Autodesk Inventor part; units mm, degrees
ref_plane "YZ Plane" through (0, 0, 0) normal (1, 0, 0) x (0, 1, 0)
ref_plane "XZ Plane" through (0, 0, 0) normal (0, 1, 0) x (-1, 0, 0)
ref_plane "XY Plane" through (0, 0, 0) normal (0, 0, 1) x (1, 0, 0)
sketch "草图1" plane through (0, 0, 0) normal (0, 0, 1) x (1, 0, 0)
  line L0 (0, 0) -> (0, 15) construction
  line L1 (2.5, 0) -> (2.5, 15)
  line L2 (-2.5, 15) -> (-2.5, 0)
  arc A0 (-2.5, 0) -> (2.5, 0) centre (0, 0) ccw
  arc A1 (2.5, 15) -> (-2.5, 15) centre (0, 15) ccw
  point P0 (0, 7.5)
  point P1 (0, -2.5)
  point P2 (0, 17.5)
  dimension "d2" = 20
  dimension "d3" = 5
extrude "拉伸1" add sketch "草图1" along normal blind 2
sketch "草图2" plane through (0, 0, 2) normal (0, 0, 1) x (1, 0, 0)
  circle A0 centre (0, 0) radius 1.5
  arc A1 (2.5, 15) -> (-2.5, 15) centre (0, 15) ccw
  circle A2 centre (0, 15) radius 1.5
  dimension "d4" = 3
  dimension "d5" = 3
extrude "拉伸2" cut sketch "草图2" against normal blind 3
properties part number "连杆2"
Part model, mm, in its own coordinate system. Coordinates: 2 decimals unless noted, no trailing zeros. Loops run counter-clockwise (first coordinate to the right, second up) from the corner with the lowest first, then second, coordinate; pieces in that order, holes last. Notation, with made-up numbers: (22.25, 11) -> (45.25, 11) arc R11 ccw to (45.25, 22) -> close; hole circle Ø6 at (84.25, 1.25). An arc over 180 degrees is marked (long way). Use a Markdown table: item, result. Add a question column.
Item 1: Band-saw the part on C-C on z = 1.3. Write the cut outline in (x, y).
Item 2: Band-saw the part on A-A on x = 0. Write the cut outline in (y, z), plus the area to 3 significant figures.
Item 3: Flat gauge pins, fed straight in: P1, Ø2.5, axis at x = 0, y = 15, coming from the -Z side; P2, Ø1, axis at x = 2, y = 9.5, coming from the -Z side; P3, Ø1, axis at x = -2, z = 0.5, coming from the +Y side. Where does each tip first touch, or does it go through?
Item 4: Probe probe 1 along Y at (x, z) = (0, 1.2); probe 2 along Y at (x, z) = (1.35, 1.05); probe 3 along X at (y, z) = (-0.5, 0.3). List the from-to ranges inside material, lowest first.
Item 5: Band-saw the part on D-D on x = -0.8. Write the cut outline in (y, z).
Item 6: Band-saw the part on B-B on y = 14.25. Write the cut outline in (x, z), plus the area to 3 significant figures.
Item 7: Pull direction Y, two halves, no side cores. Call faces 1 (the cylindrical face through (-0.1, 17.5, 1)), 2 (the flat face through (2.5, 7, 1)), 3 (the cylindrical face through (-1.5, 0.07, 1.01)): +Y half, -Y half, draft (parallel to the pull), parting line (faces both ways), or undercut.
Geometry says:
| question | item | result |
|---|---|---|
| 1 | outline | (-2.5, 0) arc R2.5 ccw to (2.5, 0) -> (2.5, 15) arc R2.5 ccw to (-2.5, 15) -> close; hole circle Ø3 at (0, 0); hole circle Ø3 at (0, 15) |
| 2 | outline | (-2.5, 0) -> (-1.5, 0) -> (-1.5, 2) -> (-2.5, 2) -> close; (1.5, 0) -> (13.5, 0) -> (13.5, 2) -> (1.5, 2) -> close; (16.5, 0) -> (17.5, 0) -> (17.5, 2) -> (16.5, 2) -> close |
| 2 | area | 28.0 mm² |
| 3 | P1 | through |
| 3 | P2 | z = 0 |
| 3 | P3 | y = 17 |
| 4 | probe 1 | -2.5 to -1.5, 1.5 to 13.5, 16.5 to 17.5 |
| 4 | probe 2 | -2.1 to -0.65, 0.65 to 14.35, 15.65 to 17.1 |
| 4 | probe 3 | -2.45 to -1.41, 1.41 to 2.45 |
| 5 | outline | (-2.37, 0) -> (-1.27, 0) -> (-1.27, 2) -> (-2.37, 2) -> close; (1.27, 0) -> (13.73, 0) -> (13.73, 2) -> (1.27, 2) -> close; (16.27, 0) -> (17.37, 0) -> (17.37, 2) -> (16.27, 2) -> close |
| 6 | outline | (-2.5, 0) -> (-1.3, 0) -> (-1.3, 2) -> (-2.5, 2) -> close; (1.3, 0) -> (2.5, 0) -> (2.5, 2) -> (1.3, 2) -> close |
| 6 | area | 4.80 mm² |
| 7 | face 1 | +Y half |
| 7 | face 2 | draft |
| 7 | face 3 | undercut |
